Geometry: see drawing. Coordinates: mm, zero at the bounding-box minimum. A direction names the side the tool comes from. Round coordinates to 2 decimals unless told otherwise and drop trailing zeros. Order: outer loops, then holes, each group sorted by start corner. A loop starts at its lowest first (then second) coordinate and runs counter-clockwise, first axis right, second up. Notation, with made-up numbers: (25, -25) -> (72, -25) arc R27 ccw to (72, -3) -> close; hole circle Ø10 at (-1, 24). An arc over 180 degrees is marked (long way). One line per item, written item: value. Start each with the question number.
1) Section B-B (y = 4). Return the cut outline in (x, z) (1 decimal).
2) Section A-A (z = 15). Return the cut outline in (x, y).
3) Section C-C (x = 34). Return the cut outline in (y, z) (1 decimal), and give its area (3 significant figures).
4) Ray query, L1, parallel to Z at x = 152, y = 9 (1 decimal); L2, parallel to X at y = 10.75, z = 26 (1 decimal); L3, parallel to X at y = 18.5, z = 37.5 (1 decimal). Return the intervals inside material, ascending.
5) Reachability of the marked faces 1 and 2 from +Z, -Z, +X, -X, +Y, -Y: full face, straight path, thin tool, end or side. Return the list, or none.
6) Pin query (flat end, axial travel): P1, Ø3, axis at x = 33, y = 7.5, coming from the +Z side; P2, Ø1, axis at x = 210.5, y = 9, coming from the -Z side; P3, Ø10, axis at y = 20, z = 8, coming from the +X side; P4, Ø10, axis at x = 102, y = 19, coming from the -Z side. Return the tip coordinate at first contact, or that it passes through.
7) Mould query, pull axis X, two halves, no side actions, for the marked faces 3 and 4. Classes: pulls with the +X half, pulls with the -X half, needs draft (parallel to the pull), parting line crosses it, or undercut.
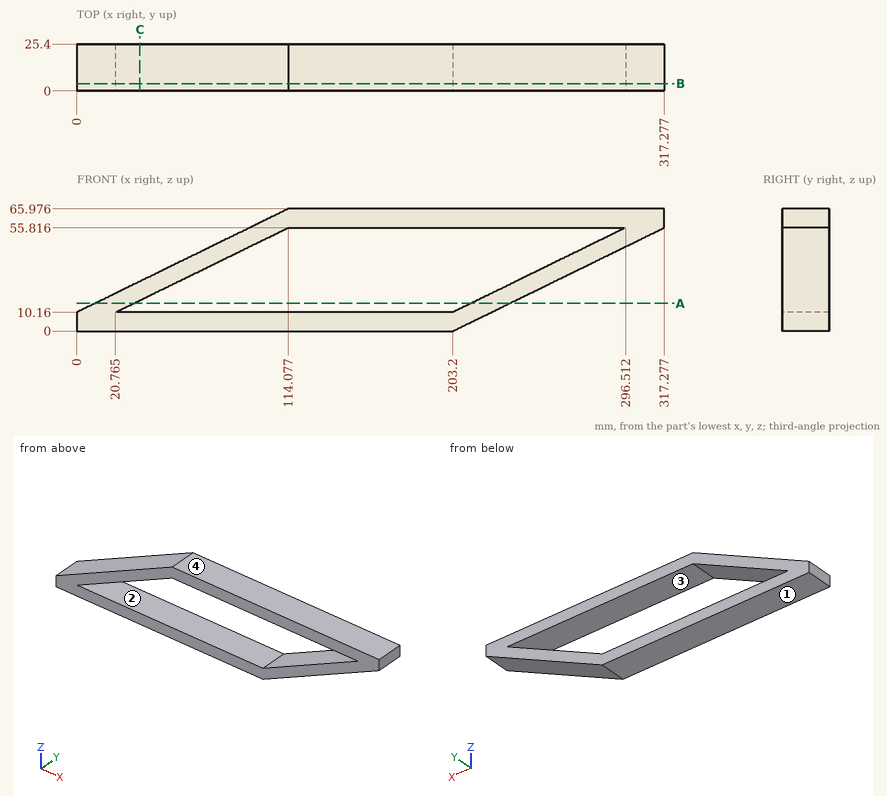
Findings:
1. outline: (0, 0) -> (203.2, 0) -> (317.3, 55.8) -> (317.3, 66) -> (114.1, 66) -> (0, 10.2) -> close; hole (20.8, 10.2) -> (203.2, 10.2) -> (296.5, 55.8) -> (114.1, 55.8) -> close
2. outline: (9.89, 0) -> (30.66, 0) -> (30.66, 25.4) -> (9.89, 25.4) -> close; (213.09, 0) -> (233.86, 0) -> (233.86, 25.4) -> (213.09, 25.4) -> close
3. outline: (0, 0) -> (25.4, 0) -> (25.4, 10.2) -> (0, 10.2) -> close; (0, 16.6) -> (25.4, 16.6) -> (25.4, 26.8) -> (0, 26.8) -> close
3. area: 516 mm2
4. L1: 0 to 10.2, 55.8 to 66
4. L2: 32.4 to 53.1, 235.6 to 256.3
4. L3: 55.9 to 76.6, 259.1 to 279.8
5. face 1: -Z, +X, -X, +Y, -Y
5. face 2: +Y, -Y
6. P1: z = 27.04
6. P2: z = 3.33
6. P3: x = 229.77
6. P4: z = 0
7. face 3: undercut
7. face 4: needs draft
